Autodesk Inventor part; units mm, degrees
ref_plane "YZ Plane" through (0, 0, 0) normal (1, 0, 0) x (0, 1, 0)
ref_plane "XZ Plane" through (0, 0, 0) normal (0, 1, 0) x (-1, 0, 0)
ref_plane "XY Plane" through (0, 0, 0) normal (0, 0, 1) x (1, 0, 0)
sketch "Sketch1" plane through (0, 0, 0) normal (0, 0, 1) x (1, 0, 0)
  line L0 (-13.429, -0.3286) -> (10.571, -0.3286)
  line L1 (-1.429, 11.6714) -> (-1.429, -12.3286)
  line L2 (5.6317, 5.6714) -> (2.571, 2.6107)
  line L3 (6.571, 5.6714) -> (6.571, 2.6714)
  line L4 (4.571, 6.7321) -> (1.5103, 3.6714)
  line L5 (-9.429, 5.6714) -> (-9.429, 2.6714)
  line L6 (-8.4897, 5.6714) -> (-5.429, 2.6107)
  line L7 (-7.429, 6.732) -> (-4.3683, 3.6714)
  line L8 (8.571, 8.6714) -> (8.571, 2.9714)
  line L9 (-11.429, 8.6714) -> (-11.429, 2.9714)
  line L10 (5.6317, -6.3286) -> (2.571, -3.2679)
  line L11 (1.871, -10.3286) -> (7.571, -10.3286)
  line L12 (-8.4897, -6.3286) -> (-5.429, -3.2679)
  line L13 (-7.429, -8.3286) -> (-4.429, -8.3286)
  line L14 (-7.429, -7.3893) -> (-4.3683, -4.3286)
  line L15 (-10.429, -10.3286) -> (-4.729, -10.3286)
  arc A0 (-11.129, -3.3286) -> (-11.429, -3.6286) centre (-11.129, -3.6286) ccw
  line L16 (-9.429, -6.3286) -> (-9.429, -3.3286)
  line L17 (-7.429, -7.3893) -> (-7.429, -8.3286)
  line L18 (-11.429, -3.6286) -> (-11.429, -9.3286)
  arc A1 (-11.429, -9.3286) -> (-10.429, -10.3286) centre (-10.429, -9.3286) ccw
  line L19 (-9.004, -10.3286) -> (-9.004, -10.3285)
  line L20 (-9.429, -6.3286) -> (-8.4897, -6.3286)
  line L21 (-11.129, -3.3286) -> (-9.429, -3.3286)
  line L22 (-11.129, 2.6714) -> (-9.429, 2.6714)
  arc A2 (-11.429, 2.9714) -> (-11.129, 2.6714) centre (-11.129, 2.9714) ccw
  arc A3 (-4.729, -10.3286) -> (-4.429, -10.0286) centre (-4.729, -10.0286) ccw
  line L23 (-4.429, -10.0286) -> (-4.429, -8.3286)
  line L24 (4.571, -7.3893) -> (4.571, -8.3286)
  line L25 (4.571, -8.3286) -> (1.571, -8.3286)
  arc A4 (1.571, -10.0286) -> (1.871, -10.3286) centre (1.871, -10.0286) ccw
  line L26 (1.571, -10.0286) -> (1.571, -8.3286)
  line L27 (4.571, -7.3893) -> (1.5103, -4.3286)
  circle A5 centre (-1.429, -0.3286) radius 2.1
  arc A6 (8.571, -3.6286) -> (8.271, -3.3286) centre (8.271, -3.6286) ccw
  line L28 (6.571, -6.3286) -> (6.571, -3.3286)
  line L29 (8.571, -3.6286) -> (8.571, -9.3286)
  arc A7 (7.571, -10.3286) -> (8.571, -9.3286) centre (7.571, -9.3286) ccw
  line L30 (5.6317, -6.3286) -> (6.571, -6.3286)
  line L31 (8.271, -3.3286) -> (6.571, -3.3286)
  line L32 (8.271, 2.6714) -> (6.571, 2.6714)
  arc A8 (8.271, 2.6714) -> (8.571, 2.9714) centre (8.271, 2.9714) ccw
  line L33 (1.871, 9.6714) -> (7.571, 9.6714)
  line L34 (-10.429, 9.6714) -> (-4.729, 9.6714)
  arc A9 (-4.429, 9.3714) -> (-4.729, 9.6714) centre (-4.729, 9.3714) ccw
  line L35 (-7.429, 7.6714) -> (-4.429, 7.6714)
  arc A10 (-10.429, 9.6714) -> (-11.429, 8.6714) centre (-10.429, 8.6714) ccw
  line L36 (-9.429, 5.6714) -> (-8.4897, 5.6714)
  line L37 (-7.429, 7.6714) -> (-7.429, 6.732)
  line L38 (-4.429, 9.3714) -> (-4.429, 7.6714)
  line L39 (1.571, 9.3714) -> (1.571, 7.6714)
  line L40 (4.571, 7.6714) -> (1.571, 7.6714)
  line L41 (4.571, 7.6714) -> (4.571, 6.7321)
  arc A11 (1.871, 9.6714) -> (1.571, 9.3714) centre (1.871, 9.3714) ccw
  arc A12 (8.571, 8.6714) -> (7.571, 9.6714) centre (7.571, 8.6714) ccw
  line L42 (5.6317, 5.6714) -> (6.571, 5.6714)
  line L43 (-5.429, 2.6107) -> (-5.429, 0.191)
  line L44 (2.571, 2.6107) -> (2.571, 0.191)
  line L45 (-4.3683, 3.6714) -> (-1.9486, 3.6714)
  line L46 (-4.3683, -4.3286) -> (-1.9486, -4.3286)
  line L47 (-1.429, 3.3714) -> (-1.9486, 3.6714)
  line L48 (-1.429, 3.3714) -> (-0.9094, 3.6714)
  line L49 (-0.9094, 3.6714) -> (1.5103, 3.6714)
  line L50 (-5.129, -0.3286) -> (-5.429, -0.8482)
  line L51 (-5.129, -0.3286) -> (-5.429, 0.191)
  line L52 (-1.429, -4.0286) -> (-0.9094, -4.3286)
  line L53 (-1.429, -4.0286) -> (-1.9486, -4.3286)
  line L54 (2.271, -0.3286) -> (2.571, 0.191)
  line L55 (2.271, -0.3286) -> (2.571, -0.8482)
  line L56 (2.571, -0.8482) -> (2.571, -3.2679)
  line L57 (-0.9094, -4.3286) -> (1.5103, -4.3286)
  line L58 (-5.429, -0.8482) -> (-5.429, -3.2679)
  point P0 (2.271, -0.3286)
  point P1 (5.6317, 5.6714)
  point P2 (8.271, 2.6714)
  point P3 (8.571, 2.9714)
  point P4 (1.871, 9.6714)
  point P5 (1.571, 9.3714)
  point P6 (-1.429, 3.3714)
  point P7 (-4.429, 9.3714)
  point P8 (-11.429, 2.9714)
  point P9 (-11.129, 2.6714)
  point P10 (-8.4897, 5.6714)
  point P11 (-5.129, -0.3286)
  point P12 (-8.4897, -6.3286)
  point P13 (-11.129, -3.3286)
  point P14 (-11.429, -3.6286)
  point P15 (-4.729, -10.3286)
  point P16 (-4.429, -10.0286)
  point P17 (-7.429, -7.3893)
  point P18 (-1.429, -4.0286)
  point P19 (4.571, -7.3893)
  point P20 (1.571, -10.0286)
  point P21 (1.871, -10.3286)
  point P22 (8.571, -3.6286)
  point P23 (8.271, -3.3286)
  point P24 (5.6317, -6.3286)
  dimension "d0" = 20
  dimension "d1" = 20
extrude "Extrusion1" add sketch "Sketch1" along normal blind 180 contours A5 L1 L48 L49 L4 L41 L40 L39 A11 L33 A12 L8 A8 L32 L3 L42 L2 L44 L54 L0 | L0 L55 L56 L10 L30 L28 L31 A6 L29 A7 L11 A4 L26 L25 L24 L27 L57 L52 L1 A5 | A5 L0 L51 L43 L6 L36 L5 L22 A2 L9 A10 L34 A9 L38 L35 L37 L7 L45 L47 L1 | L1 L53 L46 L14 L17 L13 L23 A3 L15 A1 L18 A0 L21 L16 L20 L12 L58 L50 L0 A5
properties part number "20x20_180mm"
Geometry: final body of the model. Coordinates: model frame, mm. A direction names the side the tool comes from. Round coordinates to 2 decimals unless told otherwise and drop trailing zeros.
Q1. Pin query (flat end, axial travel): P1, Ø1.2, axis at y = 1, z = 52.5, coming from the -X side. Return the tip coordinate at first contact, or that it passes through.
Q2. Pull-direction query (Y, two-part tool) for faces 1 (the flat face through (3.06, 5.22, 88.74)), 2 (the flat face through (-8, 9.671, 89)), 3 (the flat face through (-11.429, 6, 89)); classes: released by +Y, released by -Y, zero draft, split by the parting line, or undercut.
Q3. Access query for faces 4 (the flat face through (-8, -10.329, 89)), 5 (the flat face through (6.571, -5, 89)). Directions: +Z, -Z, +X, -X, +Y, -Y. A direction counts if a zero-diameter tool reaches every point of the face in a straight line with its end or side. Return the directions, or none.
Q4. Material intervals for L1, parallel to X at y = 8.5, z = 31; L2, parallel to X at y = 4.75, z = 58; L3, parallel to X at y = -4.25, z = 168.5, sorted ascending.
Evaluation:
1. P1: stops at x = -5.43
2. face 1: undercut
2. face 2: released by +Y
2. face 3: zero draft
3. face 4: +Z, -Z, +X, -X, -Y
3. face 5: +Z, -Z
4. L1: x = -11.43 to -4.43, 1.57 to 8.57
4. L2: x = -11.43 to -9.43, -7.57 to -5.45, 2.59 to 4.71, 6.57 to 8.57
4. L3: x = -11.43 to -9.43, -6.41 to -1.81, -1.05 to 3.55, 6.57 to 8.57
